from build123d import *

# Parameters (mm, degrees)
SKETCH1_R           = 9.525
BOSS_EXTRUDE1_DEPTH = 12.7
SKETCH2_W           = 20.32
SKETCH2_H           = 20.32
BOSS_EXTRUDE2_DEPTH = 7.62
CUT_EXTRUDE2_DEPTH  = 25.886815787
SKETCH5_R           = 2.000000064
CUT_EXTRUDE3_DEPTH  = 25.886815787


with BuildPart() as part:
    # Sketch1 → Boss-Extrude1 (new body)
    with BuildSketch(Plane(origin=(0, 0, 0), x_dir=(1, 0, 0), z_dir=(0, 1, 0))):
        with Locations(Location((0, 0, 0), (0, 0, 270))):
            Circle(SKETCH1_R)
    extrude(amount=BOSS_EXTRUDE1_DEPTH)

    # Sketch2 → Boss-Extrude2 (add)
    with BuildSketch(Plane(origin=(0, 12.7, 0), x_dir=(1, 0, 0), z_dir=(0, 1, 0))):
        Rectangle(SKETCH2_W, SKETCH2_H)
    extrude(amount=BOSS_EXTRUDE2_DEPTH)

    # Sketch3 → Cut-Extrude2 (cut, through all)
    with BuildSketch(Plane(origin=(0, 20.32, 0), x_dir=(1, 0, 0), z_dir=(0, 1, 0))):
        with BuildLine():
            Line((-6.506813736, 10.16), (-10.16, 10.16))
            Line((-10.16, 10.16), (-10.16, 6.506813736))
            ThreePointArc((-10.16, 6.506813736), (-8.531243315, 8.531243315), (-6.506813736, 10.16))
        make_face()
        with BuildLine():
            Line((10.16, 10.16), (6.506813736, 10.16))
            ThreePointArc((6.506813736, 10.16), (8.531243315, 8.531243315), (10.16, 6.506813736))
            Line((10.16, 6.506813736), (10.16, 10.16))
        make_face()
        with BuildLine():
            Line((10.16, -10.16), (10.16, -6.506813736))
            ThreePointArc((10.16, -6.506813736), (8.531243315, -8.531243315), (6.506813736, -10.16))
            Line((6.506813736, -10.16), (10.16, -10.16))
        make_face()
        with BuildLine():
            ThreePointArc((-6.506813736, -10.16), (-8.531243315, -8.531243315), (-10.16, -6.506813736))
            Line((-10.16, -6.506813736), (-10.16, -10.16))
            Line((-10.16, -10.16), (-6.506813736, -10.16))
        make_face()
    extrude(amount=-CUT_EXTRUDE2_DEPTH, mode=Mode.SUBTRACT)

    # Sketch5 → Cut-Extrude3 (cut, through all)
    with BuildSketch(Plane(origin=(0, 20.32, 0), x_dir=(1, 0, 0), z_dir=(0, 1, 0))):
        with Locations(Location((0, 0, 0), (0, 0, 270))):
            Circle(SKETCH5_R)
    extrude(amount=-CUT_EXTRUDE3_DEPTH, mode=Mode.SUBTRACT)


solid = part.part
The model under review builds one solid part; all positions refer to its coordinate system, in mm. A direction names the side the tool comes from. Round coordinates to 2 decimals unless told otherwise and drop trailing zeros. Loops run counter-clockwise (first coordinate to the right, second up) from the corner with the lowest first, then second, coordinate; pieces in that order, holes last. Notation, with made-up numbers: (89, 78.5) -> (140, 78.5) arc R9 cw to (140, 87.5) -> close; hole circle Ø4 at (-22, 49). An arc over 180 degrees is marked (long way). One line per question, with ' | ' between items. Start each with the question number.
Item 1: Wall thickness on line 1 along X through (y, z) = (5.25, 0) (3 decimals); line 2 along X through (y, z) = (15.25, 0); line 3 along Z through (x, y) = (0.5, 10): over which ranges is each line inside the solid? List them lowest first. Write a range as [from, to].
Item 2: Add section D-D, the plane z = 8. Write out the cut boundary in (x, y).
Item 3: Draft analysis for pull direction X (two halves, no side actions). For faces 3 (the face through (-10.16, 16, 0)), 4 (the face through (8.505, 16.563, -8.557)), 5 (the face through (0.601, 10.302, 1.908)), state which applies: +X half, -X half, draft (parallel to the pull), parting line (faces both ways), or undercut.
Item 4: Add section C-C, the plane x = 0. Write out the cut boundary in (y, z) (3 decimals).
Item 5: For pin 1 (1.5 mm diameter, centred on x = 6.5, y = 5.5, fed in from -Z); pin 2 (1.5 mm diameter, centred on y = 6, z = -7, fed in from +X), all flat-tipped, find the tip position at first contact; note any pin that passes through.
Item 6: Machinability: for faces 1 (the face through (0, 16, 10.16)), 2 (the face through (-5.796, 6.261, -7.559)), which of the approach directions +Z, -Z, +X, -X, +Y, -Y give a long, thin tool a straight path to every point of the face, cutting with its end or side? Answer none if there is none.
Item 7: Add section A-A, the plane z = 0. Write out the cut boundary in (x, y) (3 decimals).
Item 8: Add section B-B, the plane y = 18. Write out the cut boundary in (x, z) (3 decimals), then the cut area to 3 significant figures.
Return value:
1) line 1: x = [-9.525, -2], [2, 9.525] | line 2: x = [-10.16, -2], [2, 10.16] | line 3: z = [-9.51, -1.94], [1.94, 9.51]
2) outline: (-9.03, 12.7) -> (-5.17, 12.7) -> (-5.17, 0) -> (5.17, 0) -> (5.17, 12.7) -> (9.03, 12.7) -> (9.03, 20.32) -> (-9.03, 20.32) -> close
3) face 3: -X half | face 4: +X half | face 5: undercut
4) outline: (0, -9.525) -> (12.7, -9.525) -> (12.7, -10.16) -> (20.32, -10.16) -> (20.32, -2) -> (0, -2) -> close; (0, 2) -> (20.32, 2) -> (20.32, 10.16) -> (12.7, 10.16) -> (12.7, 9.525) -> (0, 9.525) -> close
5) pin 1: stops at z = -7.59 | pin 2: stops at x = 7.19
6) face 1: +Z, +X, -X, +Y, -Y | face 2: -Y
7) outline: (-10.16, 12.7) -> (-9.525, 12.7) -> (-9.525, 0) -> (-2, 0) -> (-2, 20.32) -> (-10.16, 20.32) -> close; (2, 0) -> (9.525, 0) -> (9.525, 12.7) -> (10.16, 12.7) -> (10.16, 20.32) -> (2, 20.32) -> close
8) outline: (-10.16, -6.507) arc R12.065 ccw to (-6.507, -10.16) -> (6.507, -10.16) arc R12.065 ccw to (10.16, -6.507) -> (10.16, 6.507) arc R12.065 ccw to (6.507, 10.16) -> (-6.507, 10.16) arc R12.065 ccw to (-10.16, 6.507) -> close; hole circle Ø4 at (0, 0) | area: 378 mm2
